Autodesk Inventor part; units mm, degrees
ref_plane "YZ Plane" through (0, 0, 0) normal (1, 0, 0) x (0, 1, 0)
ref_plane "XZ Plane" through (0, 0, 0) normal (0, 1, 0) x (-1, 0, 0)
ref_plane "XY Plane" through (0, 0, 0) normal (0, 0, 1) x (1, 0, 0)
sketch "Sketch1" plane through (0, 0, 0) normal (0, 1, 0) x (-1, 0, 0)
  line L0 (0, 0) -> (145, 0)
  line L1 (145, 0) -> (145, -30)
  line L2 (145, -30) -> (0, -30)
  line L3 (0, -30) -> (0, 0)
  line L4 (145, 0) -> (115, 0)
  line L5 (115, 0) -> (115, -70)
  line L6 (115, -70) -> (145, -70)
  line L7 (145, -70) -> (145, 0)
  point P0 (115, -30)
  dimension "d0" = 145
  dimension "d1" = 30
  dimension "d2" = 30
  dimension "d3" = 70
extrude "Extrusion1" add sketch "Sketch1" along normal blind 30
sketch "Sketch2" plane through (0, 0, -30) normal (0, 0, -1) x (-1, 0, 0)
  line L0 (0, 20) -> (135, 20)
  line L1 (135, 20) -> (135, 10)
  line L2 (135, 10) -> (0, 10)
  line L3 (0, 10) -> (0, 20)
  dimension "d32" = 135
  dimension "d33" = 10
extrude "Extrusion2" cut sketch "Sketch2" along normal blind 50 and the other way blind 20
sketch "Sketch4" plane through (0, 30, 0) normal (0, 1, 0) x (1, 0, 0)
  line L0 (0, 0) -> (-145, 0)
  line L1 (-145, 0) -> (-145, 10)
  line L2 (-145, 10) -> (0, 10)
  line L3 (0, 10) -> (0, 0)
  line L4 (-115, 70) -> (-145, 70)
  line L5 (-145, 70) -> (-135, 70)
  line L6 (-135, 70) -> (-135, 10)
  line L7 (-135, 10) -> (-145, 10)
  line L8 (-145, 10) -> (-145, 70)
  line L9 (-115, 30) -> (-115, 70)
  line L10 (-115, 70) -> (-125, 70)
  line L11 (-125, 70) -> (-125, 30)
  line L12 (-125, 30) -> (-115, 30)
  line L13 (-115, 30) -> (-115, 70)
  line L14 (0, 30) -> (-125, 30)
  line L15 (-125, 30) -> (-125, 20)
  line L16 (-125, 20) -> (0, 20)
  line L17 (0, 20) -> (0, 30)
  dimension "d22" = 145
  dimension "d23" = 10
  dimension "d24" = 10
  dimension "d25" = 60
  dimension "d26" = 10
  dimension "d27" = 40
  dimension "d28" = 125
  dimension "d29" = 10
extrude "Extrusion4" add sketch "Sketch4" along normal blind 20
sketch "Sketch5" plane through (0, 0, 0) normal (1, 0, 0) x (0, 0, -1)
  line L0 (0, 0) -> (0, 50)
  line L1 (30, 0) -> (30, 10)
  line L2 (0, 50) -> (30, 50)
  line L3 (30, 50) -> (30, 0)
  line L4 (30, 0) -> (0, 0)
  line L5 (0, 0) -> (0, 50)
extrude "Extrusion5" cut sketch "Sketch5" against normal blind 65
sketch "Sketch6" plane through (-115, 0, -70) normal (0, 0, -1) x (-1, 0, 0)
  line L0 (20, 10) -> (0, 10)
  line L1 (0, 0) -> (0, 10)
  line L2 (0, 0) -> (30, 0)
  line L3 (30, 0) -> (30, 50)
  line L4 (20, 50) -> (30, 50)
  line L5 (20, 30) -> (20, 50)
  line L6 (10, 30) -> (20, 30)
  line L7 (10, 30) -> (10, 50)
  line L8 (0, 50) -> (10, 50)
  line L9 (0, 20) -> (0, 50)
  line L10 (0, 20) -> (20, 20)
  line L11 (20, 20) -> (20, 10)
  point P0 (-115, 0)
extrude "Extrusion6" add sketch "Sketch6" along normal blind 10
fillet "Fillet1" radius 9.9 9 edges at (-115, 35, -30) (-115, 5, -30) (-115, 35, -80) (-115, 5, -80) (-65, 35, -30) (-65, 5, -30) (-145, 25, -80) (-65, 25, 0) (-145, 25, 0)
fillet "Fillet2" radius 2 18 edges at (-67.8996, 50, -2.8996) (-65, 50, -9.95) (-142.1004, 50, -2.8996) (-145, 50, -40) (-142.1004, 50, -77.1004) (-135.05, 50, -80) (-105, 50, 0) (-100, 50, -10) (-125, 50, -50) (-95, 50, -20) (-112.1004, 50, -32.8996) (-115, 50, -55) (-117.8996, 50, -77.1004) (-124.95, 50, -80) (-67.8996, 50, -27.1004) (-65, 50, -20.05) (-90, 50, -30) (-135, 50, -45)
properties part number "TSU_Corner1_Clamp"
The model under review builds one solid part; all positions refer to its coordinate system, in mm. A direction names the side the tool comes from. Round coordinates to 2 decimals unless told otherwise and drop trailing zeros. Loops run counter-clockwise (first coordinate to the right, second up) from the corner with the lowest first, then second, coordinate; pieces in that order, holes last. Notation, with made-up numbers: (-33.5, -31.75) -> (-8.5, -31.75) arc R17 ccw to (-8.5, -19.75) -> close; hole circle Ø8 at (40.25, 35.5). An arc over 180 degrees is marked (long way). Write item = value, one per line. Start each with the question number.
Item 1: Take a section at D-D on z = -56.5. Give the boundary of the cut face in (x, y), plus the area to 3 significant figures.
Item 2: Take a section at A-A on y = 33.5. Give the boundary of the cut face in (x, z).
Item 3: Mouldability with a two-part tool opening along X and no side actions: class faces 1 (the flat face through (-135, 39, -45)), 2 (the flat face through (-100, 39, -10)), 3 (the cylindrical face through (-67.8, 5.1, -27)) as released by +X, released by -X, zero draft, split by the parting line, or undercut.
Item 4: To check wall thickness, follow L1, parallel to X at y = 44, z = -49.5; L2, parallel to Z at x = -78, y = 40; L3, parallel to Y at x = -118, z = -25. State the ranges of each line that lie inside material, in increasing order.
Item 5: Insertion check: pin 1 (3 mm diameter, centred on y = 16.5, z = -62, fed in from +X); pin 2 (3 mm diameter, centred on y = 33.5, z = -53.5, fed in from +X); pin 3 (22.5 mm diameter, centred on x = -85, y = 29.5, fed in from -Z); pin 4 (21 mm diameter, centred on x = -103.5, z = -58.5, fed in from -Y). Each pin has a flat end and moves straight along its axis. Give the tip position at first contact, or say it passes through.
Item 6: For faces 4 (the flat face through (-115, 5, -55)), 5 (the cylindrical face through (-89.79, 49.4, -29.43)), 6 (the cylindrical face through (-95.42, 49.4, -20.57)), 7 (the flat face through (-135, 15, -45)), list the 3-axis set-ups (+Z, -Z, +X, -X, +Y, -Y) from which the entire face can be reached by the end or side of a thin tool; tool diameter is ignored.
Item 7: Take a section at B-B on x = -103.5. Give the boundary of the cut face in (y, z).
Item 8: Take a section at C-C on y = 3.5. Give the boundary of the cut face in (x, z).
Result:
q1.outline = (-145, 0) -> (-115, 0) -> (-115, 10) -> (-135, 10) -> (-135, 20) -> (-115, 20) -> (-115, 48) arc R2 ccw to (-117, 50) -> (-123, 50) arc R2 ccw to (-125, 48) -> (-125, 30) -> (-135, 30) -> (-135, 48) arc R2 ccw to (-137, 50) -> (-143, 50) arc R2 ccw to (-145, 48) -> close
q1.area = 1,100 mm²
q2.outline = (-145, -70.1) arc R9.9 ccw to (-135.1, -80) -> (-135, -80) -> (-135, -10) -> (-65, -10) -> (-65, -9.9) arc R9.9 ccw to (-74.9, 0) -> (-135.1, 0) arc R9.9 ccw to (-145, -9.9) -> close; (-125, -80) -> (-124.9, -80) arc R9.9 ccw to (-115, -70.1) -> (-115, -39.9) arc R9.9 cw to (-105.1, -30) -> (-74.9, -30) arc R9.9 ccw to (-65, -20.1) -> (-65, -20) -> (-125, -20) -> close
q3.face_1 = undercut
q3.face_2 = zero draft
q3.face_3 = released by +X
q4.L1 = -145 to -135, -125 to -115
q4.L2 = -30 to -20, -10 to 0
q4.L3 = 0 to 10, 20 to 50
q5.pin_1 = -135
q5.pin_2 = -115
q5.pin_3 = -30
q5.pin_4 = through
q6.face_4 = -Z, +X, +Y, -Y
q6.face_5 = -Z, +X, +Y
q6.face_6 = +X, +Y
q6.face_7 = -Z, +X
q7.outline = (0, -30) -> (10, -30) -> (10, -10) -> (20, -10) -> (20, -30) -> (48, -30) arc R2 ccw to (50, -28) -> (50, -22) arc R2 ccw to (48, -20) -> (30, -20) -> (30, -10) -> (48, -10) arc R2 ccw to (50, -8) -> (50, -2) arc R2 ccw to (48, 0) -> (0, 0) -> close
q8.outline = (-145, -70.1) arc R9.9 ccw to (-135.1, -80) -> (-124.9, -80) arc R9.9 ccw to (-115, -70.1) -> (-115, -39.9) arc R9.9 cw to (-105.1, -30) -> (-74.9, -30) arc R9.9 ccw to (-65, -20.1) -> (-65, -9.9) arc R9.9 ccw to (-74.9, 0) -> (-135.1, 0) arc R9.9 ccw to (-145, -9.9) -> close
